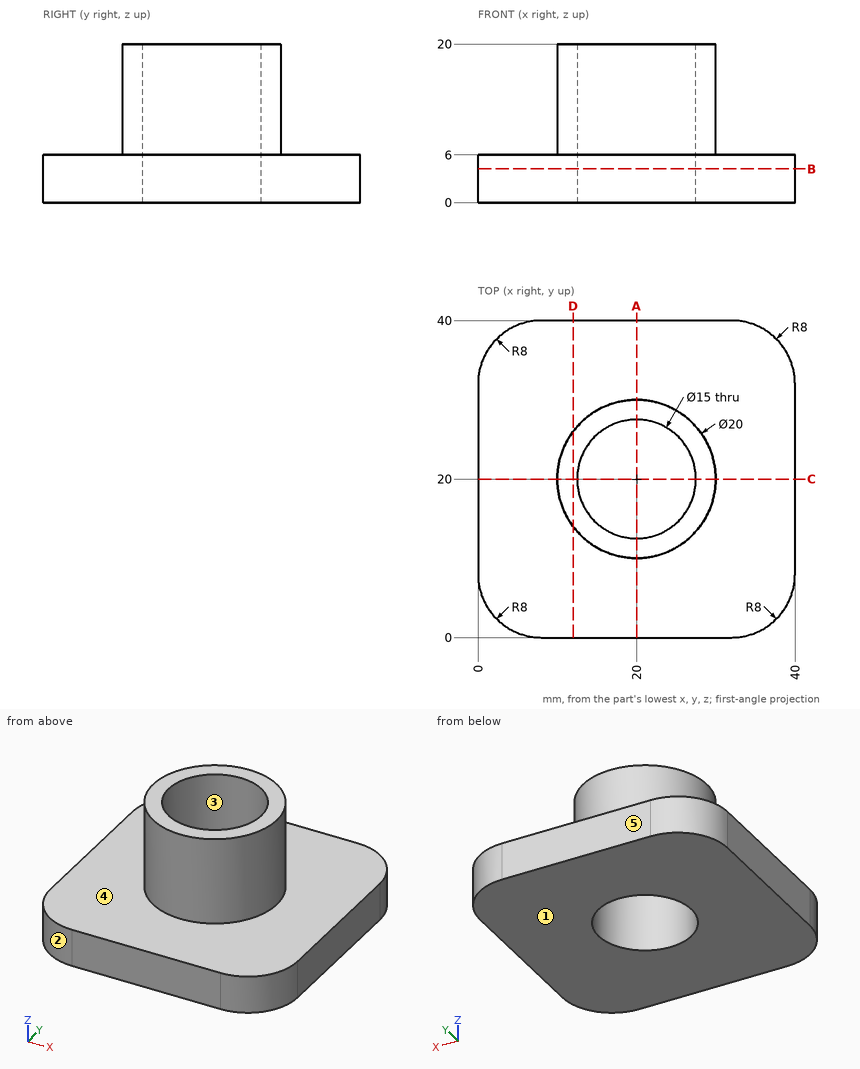
The drawing under review shows one solid part. Ordinate dimensions are in mm from its lowest x, y, z. A direction names the side the tool comes from. Round coordinates to 2 decimals unless told otherwise and drop trailing zeros. Loops run counter-clockwise (first coordinate to the right, second up) from the corner with the lowest first, then second, coordinate; pieces in that order, holes last. Notation, with made-up numbers: (-39.5, -8) - (-10.5, -8) arc R21 ccw to (-10.5, 17) - close; hole circle Ø9 at (42, 40). An arc over 180 degrees is marked (long way). Put each result on its own line as item: value. Start each with the question number.
1. Consider section A-A on x = 20. State the section outline as (y, z) points, plus the area to 3 significant figures.
2. Consider section B-B on z = 4.25. State the section outline as (x, y) points, plus the area to 3 significant figures.
3. Mouldability with a two-part tool opening along X and no side actions: class the marked faces 1, 2 and 3 as +X half, -X half, draft (parallel to the pull), parting line (faces both ways), or undercut.
4. For the marked faces 4 and 5, list the 3-axis set-ups (+Z, -Z, +X, -X, +Y, -Y) from which the entire face can be reached by the end or side of a thin tool; tool diameter is ignored.
5. Insertion check: P1, Ø1, axis at y = 21, z = 8, coming from the -X side. The pin has a flat end and moves straight along its axis. Give the tip position at first contact, or say it passes through.
6. Consider section D-D on x = 12. State the section outline as (y, z) points, plus the area to 3 significant figures.
7. For probe 1 along Y at (x, z) = (20, 5.75); probe 2 along Y at (x, z) = (20, 14.5); probe 3 along Z at (x, y) = (9.5, 14), list the stretches that pass through material, from the lowest coordinate up. Write a range as [from, to].
Result sheet:
1. outline: (0, 0) - (12.5, 0) - (12.5, 20) - (10, 20) - (10, 6) - (0, 6) - close; (27.5, 0) - (40, 0) - (40, 6) - (30, 6) - (30, 20) - (27.5, 20) - close
1. area: 220 mm^2
2. outline: (0, 8) arc R8 ccw to (8, 0) - (32, 0) arc R8 ccw to (40, 8) - (40, 32) arc R8 ccw to (32, 40) - (8, 40) arc R8 ccw to (0, 32) - close; hole circle Ø15 at (20, 20)
2. area: 1,370 mm^2
3. face 1: draft
3. face 2: -X half
3. face 3: undercut
4. face 4: +Z
4. face 5: +Z, -Z, +X, -X, +Y
5. P1: x = 10.01
6. outline: (0, 0) - (40, 0) - (40, 6) - (26, 6) - (26, 20) - (14, 20) - (14, 6) - (0, 6) - close
6. area: 408 mm^2
7. probe 1: [0, 12.5], [27.5, 40]
7. probe 2: [10, 12.5], [27.5, 30]
7. probe 3: [0, 6]
